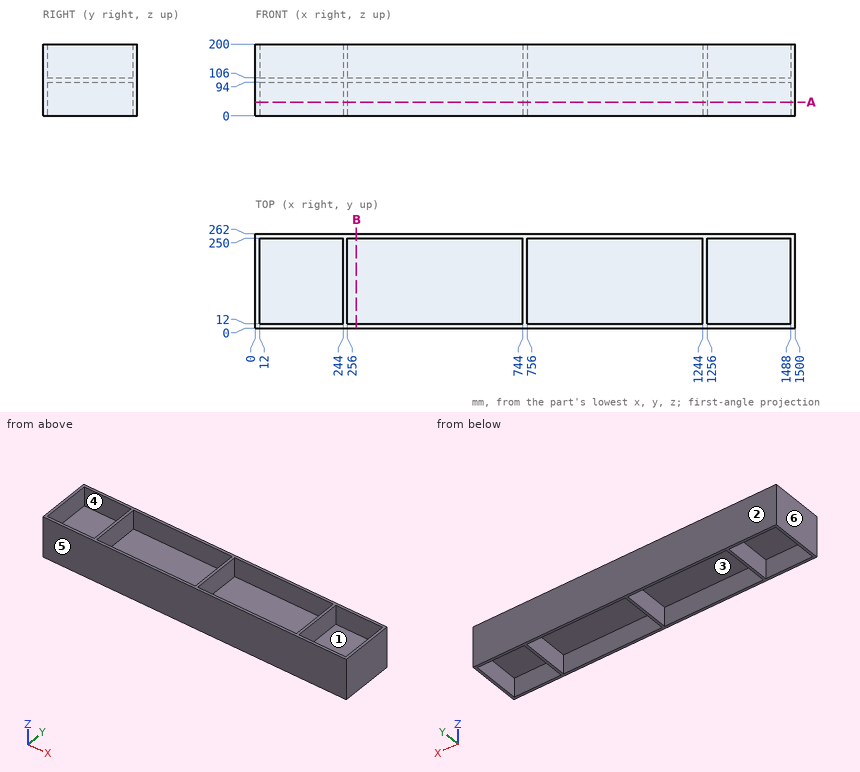
Input: dimensioned drawing with shaded views. Units: mm. Origin: part minimum x, y, z. A direction names the side the tool comes from. Coordinates: 2 decimals unless noted, no trailing zeros. Order: outer loops, then holes, each group sorted by start corner. A loop starts at its lowest first (then second) coordinate and runs counter-clockwise, first axis right, second up.
1. Ray query, line 1 along X through (y, z) = (25.5, 69.5); line 2 along Y through (x, z) = (1208.5, 107); line 3 along Z through (x, y) = (780.5, 212.5). Return the intervals inside material, ascending.
Checked values:
line 1: x = 0 to 12, 244 to 256, 744 to 756, 1244 to 1256, 1488 to 1500
line 2: y = 0 to 12, 250 to 262
line 3: z = 94 to 106
2. Draft query along X for the marked faces 4, 5 and 6. Return one class per face: +X half, -X half, draft (parallel to the pull), parting line (faces both ways), or undercut.
Checked values:
face 4: undercut
face 5: draft
face 6: -X half
3. Cut plane A-A, the plane z = 38.5. Return loops of the section in (x, y).
Checked values:
outline: (0, 0) - (1500, 0) - (1500, 262) - (0, 262) - close; hole (12, 12) - (244, 12) - (244, 250) - (12, 250) - close; hole (256, 12) - (744, 12) - (744, 250) - (256, 250) - close; hole (756, 12) - (1244, 12) - (1244, 250) - (756, 250) - close; hole (1256, 12) - (1488, 12) - (1488, 250) - (1256, 250) - close
4. Contact query for flat-ended pins moving along their axis: P1, Ø5, axis at x = 636, y = 217, coming from the -Z side; P2, Ø3, axis at x = 856, y = 117, coming from the +Z side. Output: stop coordinate, or through.
Checked values:
P1: stops at z = 94
P2: stops at z = 106
5. Access query for the marked faces 1, 2 and 3. Directions: +Z, -Z, +X, -X, +Y, -Y. A direction counts if a zero-diameter tool reaches every point of the face in a straight line with its end or side. Return the directions, or none.
Checked values:
face 1: +Z
face 2: +Z, -Z, +X, -X, +Y
face 3: -Z
6. Cut plane B-B, the plane x = 281. Return loops of the section in (y, z), plus the area to 3 significant figures.
Checked values:
outline: (0, 0) - (12, 0) - (12, 94) - (250, 94) - (250, 0) - (262, 0) - (262, 200) - (250, 200) - (250, 106) - (12, 106) - (12, 200) - (0, 200) - close
area: 7,660 mm2
